```python
from build123d import *

# Parameters (mm, degrees)
SALIENTE_EXTRUIR1_DEPTH = 5.5
CROQUIS2_W              = 15
CROQUIS2_H              = 5.5
CORTAR_EXTRUIR2_DEPTH   = 5.5


with BuildPart() as part:
    # Croquis1 → Saliente-Extruir1 (new body)
    with BuildSketch(Plane.XY):
        Polygon((27.331158202, -0.2), (27.331158202, -216.4), (-227.473920626, -216.4), (-227.473920626, -206.4), (-203.831058672, -206.4), (-203.831058672, -200.8), (-287.473920626, -200.8), (-287.473920626, -15.8), (-200, -15.8), (-200, -10.2), (-227.473920626, -10.2), (-227.473920626, -0.2), align=None)
    extrude(amount=SALIENTE_EXTRUIR1_DEPTH)

    # Croquis2 → Cortar-Extruir2 (cut)
    with BuildSketch(Plane.XY.offset(5.5)):
        with Locations((-46.837001408, -115.8)):
            Rectangle(CROQUIS2_W, CROQUIS2_H)
        with Locations((-111.837001408, -100.8)):
            Rectangle(CROQUIS2_W, CROQUIS2_H)
        with Locations((-176.837001408, -100.8)):
            Rectangle(CROQUIS2_W, CROQUIS2_H)
        with Locations((-46.837001408, -100.8)):
            Rectangle(CROQUIS2_W, CROQUIS2_H)
        with Locations((-111.837001408, -115.8)):
            Rectangle(CROQUIS2_W, CROQUIS2_H)
        with Locations((-176.837001408, -115.8)):
            Rectangle(CROQUIS2_W, CROQUIS2_H)
    extrude(amount=-CORTAR_EXTRUIR2_DEPTH, mode=Mode.SUBTRACT)


solid = part.part
```
The model under review builds one solid part; all positions refer to its coordinate system, in mm. Round coordinates to 2 decimals unless told otherwise and drop trailing zeros. Order: outer loops, then holes, each group sorted by start corner. A loop starts at its lowest first (then second) coordinate and runs counter-clockwise, first axis right, second up.
Item 1: To check wall thickness, follow probe 1 along X at (y, z) = (-118, 4.4); probe 2 along Y at (x, z) = (-214, 4.2); probe 3 along X at (y, z) = (-208, 4.05). State the ranges of each line that lie inside material, in increasing order.
Working result:
probe 1: x = -287.47 to -184.34, -169.34 to -119.34, -104.34 to -54.34, -39.34 to 27.33
probe 2: y = -216.4 to -206.4, -200.8 to -15.8, -10.2 to -0.2
probe 3: x = -227.47 to 27.33
Item 2: Add section B-B, the plane x = -238. State the section outline as (y, z) points.
Working result:
outline: (-200.8, 0) - (-15.8, 0) - (-15.8, 5.5) - (-200.8, 5.5) - close
Item 3: For pin 1 (1.6 mm diameter, centred on y = -6.5, z = 2, fed in from -X), flat-tipped, find the tip position at first contact; note if it passes through.
Working result:
pin 1: stops at x = -227.47
Item 4: Add section A-A, the plane x = -112. State the section outline as (y, z) points, and give its area (3 significant figures).
Working result:
outline: (-216.4, 0) - (-118.55, 0) - (-118.55, 5.5) - (-216.4, 5.5) - close; (-113.05, 0) - (-103.55, 0) - (-103.55, 5.5) - (-113.05, 5.5) - close; (-98.05, 0) - (-0.2, 0) - (-0.2, 5.5) - (-98.05, 5.5) - close
area: 1,130 mm2
Item 5: Add section C-C, the plane z = 2.25. Count the separate pieces of the cut face and the enclosed holes in it, and give its area (3 significant figures).
Working result:
separate pieces: 1
enclosed holes: 6
area: 65,400 mm2
